Build history of the part. All positions in model axes, mm. A direction names the side the tool comes from. Round coordinates to 2 decimals unless told otherwise and drop trailing zeros. Write each loop counter-clockwise with the first axis right and the second up, starting at its lowest first coordinate (ties: lowest second). Pieces come first, ordered by that corner, then holes.
Autodesk Inventor part; units mm, degrees
ref_plane "Combination_Module_XY" through (0, 0, 0) normal (1, 0, 0) x (0, 0, -1)
ref_plane "Combination_Module_YZ" through (0, 0, 0) normal (0, 0, -1) x (0, 1, 0)
ref_plane "Combination_Module_ZX" through (0, 0, 0) normal (0, 1, 0) x (1, 0, 0)
sketch "Sketch_1" plane through (0, 0, 0) normal (0, 0, 1) x (1, 0, 0)
  line L0 (15, 0) -> (0, 0)
  line L1 (0, 2.7) -> (0.4, 2.7)
  line L2 (0.4, 2.7) -> (0.4, 2.9)
  line L3 (0.4, 2.9) -> (0.7, 2.9)
  line L4 (0.7, 2.9) -> (0.7, 2.5)
  line L5 (0.7, 2.5) -> (14.3, 2.5)
  line L6 (14.3, 2.5) -> (14.3, 2.9)
  line L7 (14.3, 2.9) -> (14.6, 2.9)
  line L8 (14.6, 2.9) -> (14.6, 2.7)
  line L9 (14.6, 2.7) -> (15, 2.7)
  line L10 (15, 2.7) -> (15, 4.5)
  arc A0 (15, 4.5) -> (14.5, 5) centre (14.5, 4.5) ccw
  line L11 (14.5, 5) -> (5, 5)
  line L12 (5, 5) -> (5, 12.65)
  line L13 (5, 12.65) -> (4.65, 13)
  line L14 (4.65, 13) -> (0.35, 13)
  line L15 (0.35, 13) -> (0, 12.65)
  line L16 (0, 12.65) -> (0, 2.7)
revolve "Revolution1" add sketch "Sketch_1" angle 360 about axis through (15, 0, 0) along (1, 0, 0)
sketch "Sketch2" plane through (0, 0, 0) normal (-1, 0, 0) x (0, 0, 1)
  point P0 (0, 9)
hole "Hole1" at (0, 9, 0) direction (1, 0, 0) diameter 3.5 depth 5 counterbore diameter 6 counterbore depth 3.1
sketch "Sketch3" plane through (0, 0, 0) normal (-1, 0, 0) x (0, 0, 1)
  point P0 (0, -9)
hole "Hole2" at (0, -9, 0) direction (1, 0, 0) diameter 3.5 depth 5 counterbore diameter 6 counterbore depth 3.1
sketch "Sketch4" plane through (0, 0, 0) normal (-1, 0, 0) x (0, 0, 1)
  point P0 (-9, 0)
hole "Hole3" at (0, 0, -9) direction (1, 0, 0) diameter 3.5 depth 5 counterbore diameter 6 counterbore depth 3.1
sketch "Sketch5" plane through (0, 0, 0) normal (-1, 0, 0) x (0, 0, 1)
  point P0 (9, 0)
hole "Hole4" at (0, 0, 9) direction (1, 0, 0) diameter 3.5 depth 5 counterbore diameter 6 counterbore depth 3.1
ref_plane "Combination_Module_XY" through (0, 0, 0) normal (1, 0, 0) x (0, 0, -1)
ref_plane "Combination_Module_YZ" through (0, 0, 0) normal (0, 0, -1) x (0, 1, 0)
ref_plane "Combination_Module_ZX" through (0, 0, 0) normal (0, 1, 0) x (1, 0, 0)
properties part number "C-LHFR5"
1) Slice it at B-B (z = 0). Count the separate pieces of the cut face and the enclosed holes in it, plus the area to 3 significant figures.
Results:
separate pieces: 4
enclosed holes: 0
area: 103 mm2
2) Which spindle directions (+Z, -Z, +X, -X, +Y, -Y) get a long thin tool onto all of the face, cutting with end or side? Do faces 1 (the cylindrical face through (14.45, -2.14, 1.96)), 2 (the cylindrical face through (14.803, -0.585, -2.636)), 3 (the flat face through (3.1, 0, 11)). Say none if no direction does.
Results:
face 1: none
face 2: +X
face 3: -X
3) Wall check: L1, parallel to Z at x = 2, y = 0; L2, parallel to Z at x = 14.45, y = 0; L3, parallel to X at y = -0.5, z = -7. Give the ranges that are in metal, low to high.
Results:
L1: z = -13 to -12, -6 to -2.5, 2.5 to 6, 12 to 13
L2: z = -5 to -2.9, 2.9 to 5
L3: x = 3.1 to 5
4) Pin check, flat tips, straight feed: pin 1 Ø1 at (x, y) = (7.5, -6) entering from +Z; pin 2 Ø3 at (y, z) = (-8, 9.5) entering from +X; pin 3 Ø3 at (y, z) = (-1, 0.5) entering from +X; pin 4 Ø6 at (x, y) = (13, 5.5) entering from -Z. Stop position of each tip, or through.
Results:
pin 1: passes through
pin 2: stops at x = 5
pin 3: stops at x = 14.3
pin 4: stops at z = -4.33
5) Slice it at A-A (x = 2.5). Write the cut outline in (y, z).
Results:
outline: circle Ø26 at (0, 0); hole circle Ø6 at (-9, 0); hole circle Ø6 at (0, -9); hole circle Ø6 at (0, 9); hole circle Ø5 at (0, 0); hole circle Ø6 at (9, 0)
6) Mould opens along Z. For faces 4 (the cylindrical face through (2.47, -10.316, 7.91)), 5 (the flat face through (5, 5.4, 0.2)), 6 (the cylindrical face through (2, -9, -3)) say: released by +Z, released by -Z, zero draft, split by the parting line, or undercut.
Results:
face 4: split by the parting line
face 5: zero draft
face 6: undercut
7) Slice it at D-D (x = 12.75). Write the cut outline in (y, z).
Results:
outline: circle Ø10 at (0, 0); hole circle Ø5 at (0, 0)
